Design review of the part built by this model. Coordinates are the model's own, in mm. Face numbers are marked on the shaded views. A direction names the side the tool comes from. Give positions to 0.01 mm unless a question says otherwise; leave off trailing zeros. Loops run counter-clockwise (first coordinate to the right, second up) from the corner with the lowest first, then second, coordinate; pieces in that order, holes last. Notation, with made-up numbers: (26, 14.5) -> (79, 14.5) arc R35 ccw to (79, 50.5) -> close; hole circle Ø4 at (58, 64.5). An arc over 180 degrees is marked (long way). Answer in a Markdown table with one row per item. Add a question column.
(1) Consider section D-D on x = -5.5. Write out the cut boundary in (y, z).
(2) For line 1 (Y direction, x = 7, z = -1.25); line 2 (X direction, y = -13.5, z = 7); line 3 (Z direction, x = -4.5, y = 1), list the stretches that pass through material, from the lowest coordinate up.
(3) For the marked faces 4, 5 and 6, list the 3-axis set-ups (+Z, -Z, +X, -X, +Y, -Y) from which the entire face can be reached by the end or side of a thin tool; tool diameter is ignored.
(4) Consider section A-A on z = 6.75. Write out the cut boundary in (x, y).
(5) Consider section B-B on x = 0. Write out the cut boundary in (y, z), then the cut area to 3 significant figures.
(6) Draft analysis for pull direction X (two halves, no side actions). For the marked faces 1, 2 and 3, state which applies: +X half, -X half, draft (parallel to the pull), parting line (faces both ways), or undercut.
(7) Consider section C-C on y = 27. Write out the cut boundary in (x, z).
(8) For pin 1 (7.5 mm diameter, centred on x = -0.5, y = 4, fed in from -Z); pin 2 (1 mm diameter, centred on y = 20.5, z = -0.5, fed in from +X), all flat-tipped, find the tip position at first contact; note any pin that passes through.
from build123d import *

# Parameters (mm, degrees)
F1_DEPTH    = 37.5
F2_T        = 2.5
F2_T3_DEPTH = 80
F4_DEPTH    = 2.5


# Not quite as in the source:
# - a shell that OpenCascade refuses in one call is made with other operations: the cavity is built on its own and cut out


with BuildPart() as f1:
    # F0 (on Front) → F1 (new body, symmetric)
    with BuildSketch(Plane.XZ):
        Polygon((-20, -3), (20, -3), (16.5358983849, 3), (22.5358983849, 3), (22.5358983849, 8), (-22.5358983849, 8), (-22.5358983849, 3), (-16.5358983849, 3), align=None)
    extrude(amount=F1_DEPTH, both=True)

    # F2: shell of thickness 2.5, made by hand


with BuildPart() as f2_core1:
    # F2_t2: copy of F1
    add(f1.part)

    # the walls: a layer under each face that stays
    f2_faces = [f2_core1.faces().sort_by_distance(p)[0] for p in [
        (-18.2679491924, 0, 0),
        (-19.5358983849, 0, 3),
        (-22.5358983849, 0, 5.5),
        (0, 0, 8),
        (22.5358983849, 0, 5.5),
        (19.5358983849, 0, 3),
        (18.2679491924, 0, 0),
        (0, -37.5, 2.5),
        (0, 37.5, 2.5),
    ]]
    thicken(f2_faces, amount=-F2_T, mode=Mode.SUBTRACT)

    # F2_s4 → F2_t3 (cut)
    with BuildSketch(Plane.XZ.offset(-40)):
        Polygon((-16.55754902, 2.9875), (-14.3708348754, 1.75), (-12.2057713659, 5.5), (-16.5358983849, 5.5), align=None)
        Polygon((16.55754902, 2.9875), (16.5358983849, 5.5), (12.2057713659, 5.5), (14.3708348754, 1.75), align=None)
    extrude(amount=F2_T3_DEPTH, mode=Mode.SUBTRACT)


with BuildPart() as f1_1:
    add(f1.part)

    # what is left inside the walls is the cavity
    f2_cavity = [f2_core1.part.solids().sort_by_distance(p)[0] for p in [
        (0, 11.666667, -2.975),
    ]]
    add(f2_cavity, mode=Mode.SUBTRACT)

    # F3 (on face) → F4 (cut, through all)
    with BuildSketch(Plane(origin=(0, 0, 5.5), x_dir=(1, 0, 0), z_dir=(0, 0, -1))):
        with BuildLine():
            Line((3, -20), (3, 20))
            ThreePointArc((3, 20), (0, 23), (-3, 20))
            Line((-3, 20), (-3, -20))
            ThreePointArc((-3, -20), (0, -23), (3, -20))
        make_face()
    extrude(amount=-F4_DEPTH, mode=Mode.SUBTRACT)


solid = f1_1.part
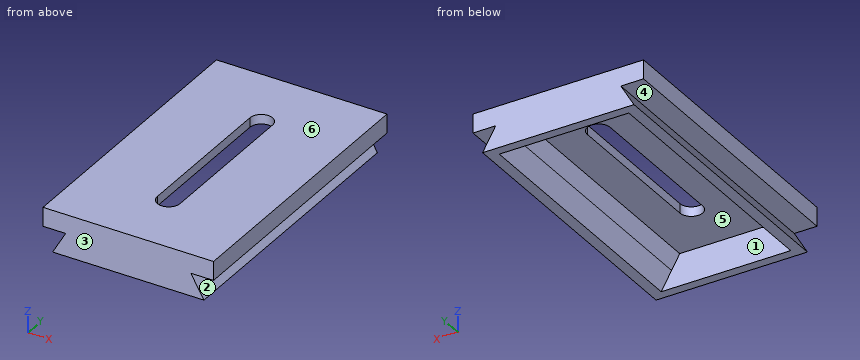
Values follow:
| question | item | result |
|---|---|---|
| 1 | outline | (-37.5, -3) -> (-35, -3) -> (-35, 5.5) -> (35, 5.5) -> (35, -3) -> (37.5, -3) -> (37.5, 8) -> (-37.5, 8) -> close |
| 2 | line 1 | -37.5 to -35, 35 to 37.5 |
| 2 | line 2 | -22.54 to -3, 3 to 22.54 |
| 2 | line 3 | 5.5 to 8 |
| 3 | face 4 | -X, +Y, -Y |
| 3 | face 5 | -Z |
| 3 | face 6 | +Z, +X, -X, +Y, -Y |
| 4 | outline | (-22.54, -37.5) -> (22.54, -37.5) -> (22.54, 37.5) -> (-22.54, 37.5) -> close; hole (-3, -20) arc R3 ccw to (3, -20) -> (3, 20) arc R3 ccw to (-3, 20) -> close |
| 5 | outline | (-37.5, -3) -> (-35, -3) -> (-35, 5.5) -> (-23, 5.5) -> (-23, 8) -> (-37.5, 8) -> close; (23, 5.5) -> (35, 5.5) -> (35, -3) -> (37.5, -3) -> (37.5, 8) -> (23, 8) -> close |
| 5 | area | 115 mm2 |
| 6 | face 1 | undercut |
| 6 | face 2 | +X half |
| 6 | face 3 | draft |
| 7 | outline | (-22.54, 3) -> (-16.54, 3) -> (-20, -3) -> (-17.11, -3) -> (-12.21, 5.5) -> (12.21, 5.5) -> (17.11, -3) -> (20, -3) -> (16.54, 3) -> (22.54, 3) -> (22.54, 8) -> (-22.54, 8) -> close |
| 8 | pin 1 | z = 5.5 |
| 8 | pin 2 | x = 18.85 |
